Verification items for the finished model (mm, model axes). Round coordinates to 2 decimals unless told otherwise and drop trailing zeros. Order: outer loops, then holes, each group sorted by start corner. A loop starts at its lowest first (then second) coordinate and runs counter-clockwise, first axis right, second up. Notation, with made-up numbers: M 53.25,29.25 L 63.25,29.25 A9 cw 63.25,45.25 Z; hole C 49.25,21 d3. An arc over 180 degrees is marked long. Answer as a JSON object with one key per item and string values. Group by question number.
```python
from build123d import *

# Parameters (mm, degrees)
SKETCH1_W           = 255
SKETCH1_H           = 130
SKETCH1_R           = 1.6
SKETCH1_R_2         = 1.1
SKETCH1_R_3         = 2.1
SKETCH1_W_2         = 10
SKETCH1_H_2         = 25
BOSS_EXTRUDE1_DEPTH = 3
FILLET1_R           = 5


with BuildPart() as part:
    # Sketch1 → Boss-Extrude1 (new body)
    with BuildSketch(Plane(origin=(0, 0, 0), x_dir=(1, 0, 0), z_dir=(0, 1, 0))):
        Rectangle(SKETCH1_W, SKETCH1_H)
        with Locations((120, -40)):
            Circle(SKETCH1_R, mode=Mode.SUBTRACT)
        with Locations((-120, -40)):
            Circle(SKETCH1_R, mode=Mode.SUBTRACT)
        with Locations((120, 40)):
            Circle(SKETCH1_R, mode=Mode.SUBTRACT)
        with Locations((-120, 40)):
            Circle(SKETCH1_R, mode=Mode.SUBTRACT)
        with Locations((32, -58)):
            Circle(SKETCH1_R_2, mode=Mode.SUBTRACT)
        with Locations((108, -58)):
            Circle(SKETCH1_R_2, mode=Mode.SUBTRACT)
        with Locations((108, 58)):
            Circle(SKETCH1_R_2, mode=Mode.SUBTRACT)
        with Locations((32, 58)):
            Circle(SKETCH1_R_2, mode=Mode.SUBTRACT)
        with Locations((-100.25, 47.25)):
            Circle(SKETCH1_R_2, mode=Mode.SUBTRACT)
        with Locations((6.25, 47.25)):
            Circle(SKETCH1_R_2, mode=Mode.SUBTRACT)
        with Locations((-100.25, -47.25)):
            Circle(SKETCH1_R_2, mode=Mode.SUBTRACT)
        with Locations((6.25, -47.25)):
            Circle(SKETCH1_R_2, mode=Mode.SUBTRACT)
        with Locations((-109.5, 0)):
            Circle(SKETCH1_R_3, mode=Mode.SUBTRACT)
        with Locations((18, 0)):
            Rectangle(SKETCH1_W_2, SKETCH1_H_2, mode=Mode.SUBTRACT)
    extrude(amount=BOSS_EXTRUDE1_DEPTH)

    # Fillet1
    fillet1_edges = [part.edges().sort_by_distance(p)[0] for p in [
        (127.5, 1.5, 65),
        (-127.5, 1.5, 65),
        (-127.5, 1.5, -65),
        (127.5, 1.5, -65),
    ]]
    fillet(fillet1_edges, radius=FILLET1_R)


solid = part.part
```
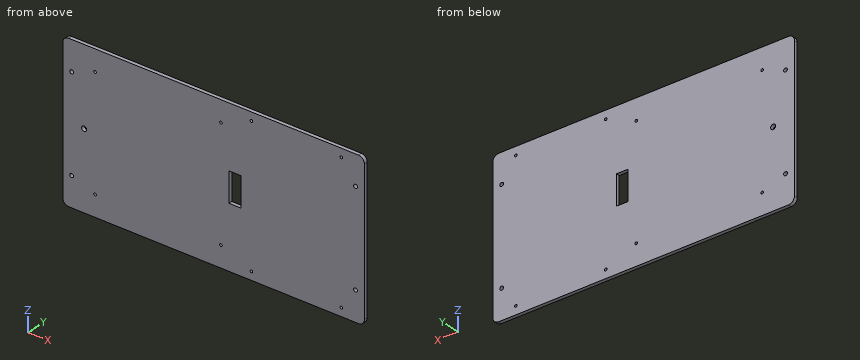
Q1. Gauge pin test, flat end, axial feed: pin 1 Ø2.5 at (x, z) = (120, 40) entering from -Y. Record the tip position at first contact, or that the pin passes through.
Q2. Cross-section at B-B, the plane x = 18. Record the cut outline in (y, z).
Q3. Cross-section at A-A, the plane z = 7. Record the cut outline in (x, y), then the cut area to 3 significant figures.
Q4. Thickness scan on line 1 (X direction, y = 1.3, z = -47.25); line 2 (Z direction, x = -100.25, y = 1.7); line 3 (Z direction, x = 120, y = 1.75). Record the ranges inside material, lowest first. Write a range as from..to.
Conclusion:
{
 "1": {"pin 1": "through"},
 "2": {"outline": "M 0,-65 L 3,-65 L 3,-12.5 L 0,-12.5 Z; M 0,12.5 L 3,12.5 L 3,65 L 0,65 Z"},
 "3": {"outline": "M -127.5,0 L 13,0 L 13,3 L -127.5,3 Z; M 23,0 L 127.5,0 L 127.5,3 L 23,3 Z", "area": "735 mm2"},
 "4": {"line 1": "-127.5..-101.35, -99.15..5.15, 7.35..127.5", "line 2": "-65..-48.35, -46.15..46.15, 48.35..65", "line 3": "-65..-41.6, -38.4..38.4, 41.6..65"}
}
